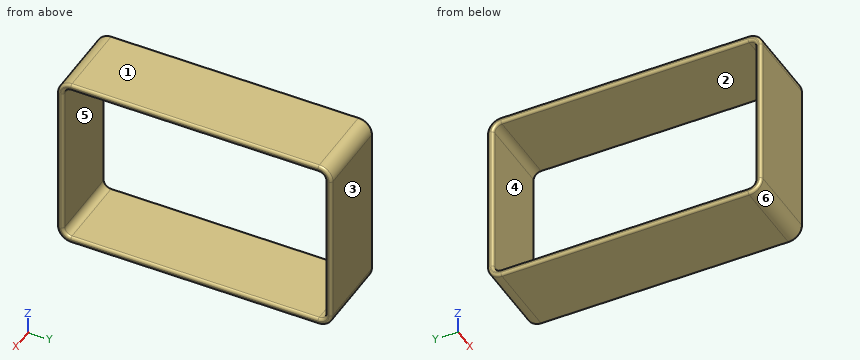
```python
from build123d import *


with BuildPart() as part:
    # Sweep1: sweep along a path in Sketch1
    with BuildLine(Plane(origin=(0, 0, 0), x_dir=(0, 0, -1), z_dir=(1, 0, 0))) as sweep1_path:
        Line((14.5, 25.5), (-14.5, 25.5))
        ThreePointArc((-14.5, 25.5), (-15.914213562, 24.914213562), (-16.5, 23.5))
        Line((-16.5, 23.5), (-16.5, -23.5))
        ThreePointArc((-16.5, -23.5), (-15.914213562, -24.914213562), (-14.5, -25.5))
        Line((-14.5, -25.5), (14.5, -25.5))
        ThreePointArc((14.5, -25.5), (15.914213562, -24.914213562), (16.5, -23.5))
        Line((16.5, -23.5), (16.5, 23.5))
        ThreePointArc((16.5, 23.5), (15.914213562, 24.914213562), (14.5, 25.5))
    # Sketch2 → Sweep1 (sweep)
    with BuildSketch(Plane.XY):
        with BuildLine():
            Line((-7, 26.1), (7, 26.1))
            ThreePointArc((7, 26.1), (7.353553391, 25.953553391), (7.5, 25.6))
            Line((7.5, 25.6), (7.5, 25.4))
            ThreePointArc((7.5, 25.4), (7.353553391, 25.046446609), (7, 24.9))
            Line((7, 24.9), (-7, 24.9))
            ThreePointArc((-7, 24.9), (-7.353553391, 25.046446609), (-7.5, 25.4))
            Line((-7.5, 25.4), (-7.5, 25.6))
            ThreePointArc((-7.5, 25.6), (-7.353553391, 25.953553391), (-7, 26.1))
        make_face()
    sweep(path=sweep1_path.line)


solid = part.part
```
The listing builds one solid part. Answer for the finished solid, in the listing's coordinates (mm). Face numbers are marked on the shaded views. A direction names the side the tool comes from. Round coordinates to 2 decimals unless told otherwise and drop trailing zeros. Loops run counter-clockwise (first coordinate to the right, second up) from the corner with the lowest first, then second, coordinate; pieces in that order, holes last.
1) A cutting plane is placed at C-C on x = 1.5. Determine the outline of the cut face in (y, z).
Outcome:
outline: (-26.1, -14.5) arc R2.6 ccw to (-23.5, -17.1) - (23.5, -17.1) arc R2.6 ccw to (26.1, -14.5) - (26.1, 14.5) arc R2.6 ccw to (23.5, 17.1) - (-23.5, 17.1) arc R2.6 ccw to (-26.1, 14.5) - close; hole (-24.9, -14.5) arc R1.4 ccw to (-23.5, -15.9) - (23.5, -15.9) arc R1.4 ccw to (24.9, -14.5) - (24.9, 14.5) arc R1.4 ccw to (23.5, 15.9) - (-23.5, 15.9) arc R1.4 ccw to (-24.9, 14.5) - close
2) Consider line 1 (Y direction, x = 3.5, z = 13); line 2 (Z direction, x = -5, y = 9); line 3 (Y direction, x = 4.75, z = -15). Determine where each line is inside the solid, lowest interval first.
Outcome:
line 1: y = -26.1 to -24.9, 24.9 to 26.1
line 2: z = -17.1 to -15.9, 15.9 to 17.1
line 3: y = -26.05 to -24.81, 24.81 to 26.05
3) For the marked faces 5 and 6, determine the directions among +Z, -Z, +X, -X, +Y, -Y from which every point of the face is accessible in a straight line to the end or side of a thin tool.
Outcome:
face 5: +X, -X
face 6: -Z, +X, -X, -Y
4) A cutting plane is placed at A-A on z = 8.5. Determine the outline of the cut face in (x, y), plus the area to 3 significant figures.
Outcome:
outline: (-7.5, -25.6) arc R0.5 ccw to (-7, -26.1) - (7, -26.1) arc R0.5 ccw to (7.5, -25.6) - (7.5, -25.4) arc R0.5 ccw to (7, -24.9) - (-7, -24.9) arc R0.5 ccw to (-7.5, -25.4) - close; (-7.5, 25.4) arc R0.5 ccw to (-7, 24.9) - (7, 24.9) arc R0.5 ccw to (7.5, 25.4) - (7.5, 25.6) arc R0.5 ccw to (7, 26.1) - (-7, 26.1) arc R0.5 ccw to (-7.5, 25.6) - close
area: 35.6 mm2
5) For a pull along Z with two mould halves and no side action, classify the marked faces 1, 2, 3 and 4 as released by +Z, released by -Z, zero draft, split by the parting line, or undercut.
Outcome:
face 1: released by +Z
face 2: undercut
face 3: zero draft
face 4: undercut
6) A cutting plane is placed at B-B on y = 15. Determine the outline of the cut face in (x, z), plus the area to 3 significant figures.
Outcome:
outline: (-7.5, -16.6) arc R0.5 ccw to (-7, -17.1) - (7, -17.1) arc R0.5 ccw to (7.5, -16.6) - (7.5, -16.4) arc R0.5 ccw to (7, -15.9) - (-7, -15.9) arc R0.5 ccw to (-7.5, -16.4) - close; (-7.5, 16.4) arc R0.5 ccw to (-7, 15.9) - (7, 15.9) arc R0.5 ccw to (7.5, 16.4) - (7.5, 16.6) arc R0.5 ccw to (7, 17.1) - (-7, 17.1) arc R0.5 ccw to (-7.5, 16.6) - close
area: 35.6 mm2
7) Given P1, Ø6, axis at y = 7.5, z = 10, coming from the +X side, flat-ended and moving along its own axis, determine where the tip first touches the part or whether it passes through.
Outcome:
P1: passes through
